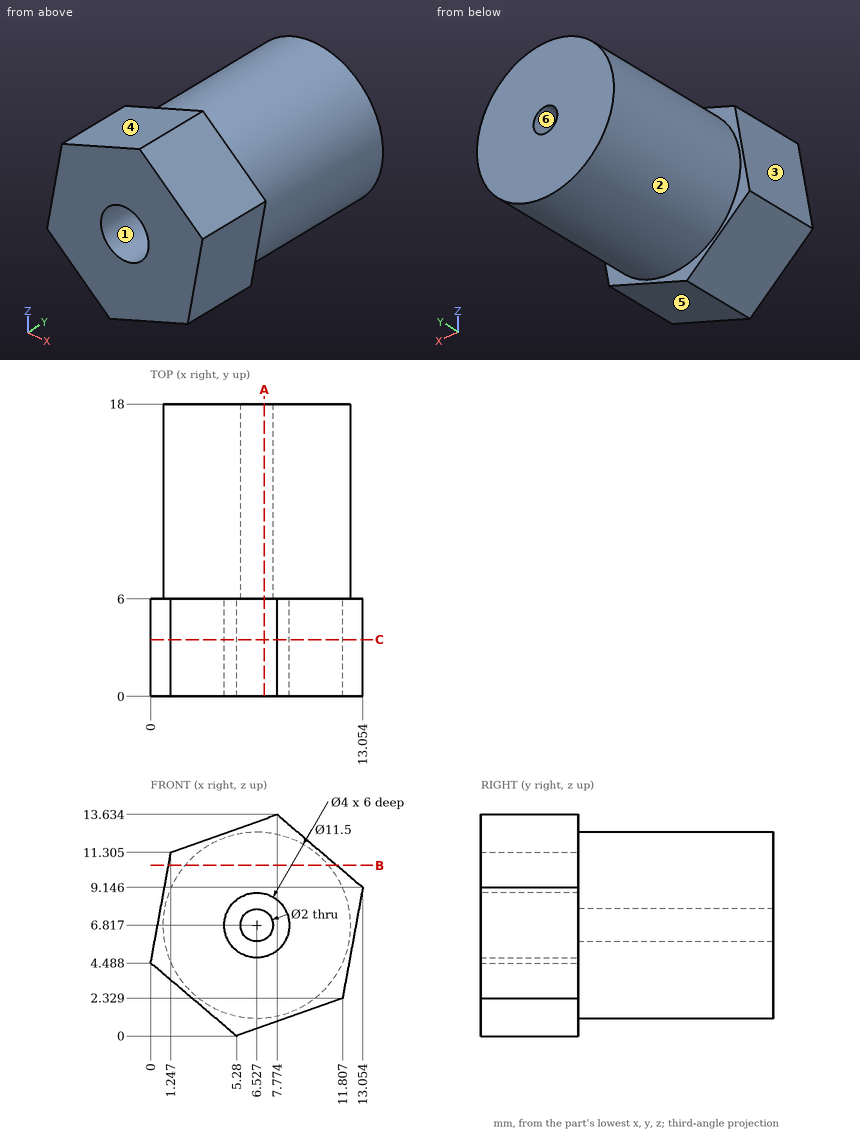
Here's the drawing with two shaded views (mm, measured from the low corner). I have some questions. A direction names the side the tool comes from. Coordinates: 2 decimals unless noted, no trailing zeros. Loops run counter-clockwise (first coordinate to the right, second up) from the corner with the lowest first, then second, coordinate; pieces in that order, holes last.
Item 1: I'm going to push flat-ended pins straight in: pin 1 (8 mm diameter, centred on y = 4, z = 9.5, fed in from -X) (1 decimal); pin 2 (2 mm diameter, centred on x = 6.5, y = 7.5, fed in from -Z); pin 3 (3 mm diameter, centred on x = 6.53, z = 6.82, fed in from -Y). Where does each tip first touch, or does it pass through?
Answers below:
pin 1: stops at x = 0.2
pin 2: stops at z = 1.07
pin 3: stops at y = 6
Item 2: Suppose I cut it at C-C (y = 3.5). Please give me the cut outline in (x, z) (1 decimal).
Answers below:
outline: (0, 4.5) - (5.3, 0) - (11.8, 2.3) - (13.1, 9.1) - (7.8, 13.6) - (1.2, 11.3) - close; hole circle Ø4 at (6.5, 6.8)
Item 3: If we mould it in two halves opening along Z, with no side actions, what happens to the marked faces 4, 5 and 6? For each: released by +Z, released by -Z, zero draft, split by the parting line, or undercut.
Answers below:
face 4: released by +Z
face 5: released by -Z
face 6: undercut
Item 4: Please list where these lines run through material, in increasing order: L1, parallel to Z at x = 7.25, y = 8.75 (1 decimal); L2, parallel to Z at x = 7.75, y = 3 (1 decimal); L3, parallel to X at y = 4.25, z = 7.75 (1 decimal).
Answers below:
L1: z = 1.1 to 6.1, 7.5 to 12.5
L2: z = 0.9 to 5.2, 8.4 to 13.6
L3: x = 0.6 to 4.8, 8.3 to 12.8
Item 5: Suppose I cut it at B-B (z = 10.5). Please give me the cut outline in (x, y).
Answers below:
outline: (1.1, 0) - (11.46, 0) - (11.46, 6) - (10.94, 6) - (10.94, 18) - (2.11, 18) - (2.11, 6) - (1.1, 6) - close
Item 6: Which directions (+Z, -Z, +X, -X, +Y, -Y) give clear straight access to the entire face, cutting with the end or side of a thin tool? Please do the marked faces 1, 2 and 3.
Answers below:
face 1: -Y
face 2: +Y
face 3: +Z, -X, +Y, -Y
Item 7: Suppose I cut it at A-A (x = 7). Please give me the cut outline in (y, z).
Answers below:
outline: (0, 0.61) - (6, 0.61) - (6, 1.09) - (18, 1.09) - (18, 5.94) - (6, 5.94) - (6, 4.87) - (0, 4.87) - close; (0, 8.76) - (6, 8.76) - (6, 7.7) - (18, 7.7) - (18, 12.55) - (6, 12.55) - (6, 13.36) - (0, 13.36) - close
